```python
from build123d import *

# Parameters (mm, degrees)
SKETCH002_W    = 80.8
SKETCH002_H    = 36
PAD001_DEPTH   = 70
THICKNESS001_T = -0.8
FILLET_R       = 1
FILLET005_R    = 0.5


with BuildPart() as part:
    # Sketch002 → Pad001 (new body)
    with BuildSketch(Plane.XY):
        Rectangle(SKETCH002_W, SKETCH002_H)
    extrude(amount=PAD001_DEPTH)

    # Thickness001
    thickness001_openings = [part.faces().sort_by_distance(p)[0] for p in [
        (0, 0, 0),
    ]]
    offset(amount=THICKNESS001_T, openings=thickness001_openings, kind=Kind.INTERSECTION)

    # Fillet
    fillet_edges = [part.edges().sort_by_distance(p)[0] for p in [
        (-40.4, 18, 35),
        (-40.4, -18, 35),
        (40.4, 18, 35),
        (0, 18, 70),
        (40.4, -18, 35),
        (40.4, 0, 70),
        (0, -18, 70),
        (-40.4, 0, 70),
    ]]
    fillet(fillet_edges, radius=FILLET_R)

    # Fillet005
    fillet005_edges = [part.edges().sort_by_distance(p)[0] for p in [
        (0, -17.2, 0),
        (-39.6, 0, 0),
        (39.6, 0, 0),
        (0, 17.2, 0),
    ]]
    fillet(fillet005_edges, radius=FILLET005_R)


with BuildPart() as part_1:
    # Body001 placement: moved
    add(part.part.moved(Location((0, 0, 127))))


solid = part_1.part
```
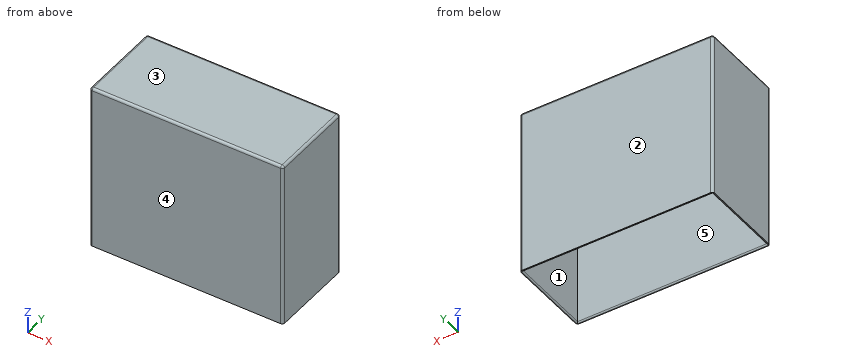
Build history of the part. All positions in model axes, mm. Face numbers are marked on the shaded views. A direction names the side the tool comes from. Round coordinates to 2 decimals unless told otherwise and drop trailing zeros. Write each loop counter-clockwise with the first axis right and the second up, starting at its lowest first coordinate (ties: lowest second). Pieces come first, ordered by that corner, then holes.
1) Pin check, flat tips, straight feed: pin 1 (6 mm diameter, centred on x = 9.5, y = 14.5, fed in from -Z); pin 2 (17 mm diameter, centred on x = -13, y = -2.5, fed in from -Z). Stop position of each tip, or through.
2) Band-saw the part on A-A, the plane y = 0. List the corners of the cut face in (x, z), and give its area (3 significant figures).
3) Mould opens along Y. For the marked faces 1, 2 and 3 say: +Y half, -Y half, draft (parallel to the pull), parting line (faces both ways), or undercut.
4) Drill centre lines: probe 1 along Y at (x, z) = (25.5, 180); probe 2 along X at (y, z) = (1, 152); probe 3 along Z at (x, y) = (2, -11). Where is each one in solid material? Low to high.
5) Band-saw the part on C-C, the plane x = -16. List the corners of the cut face in (y, z).
6) Band-saw the part on B-B, the plane z = 189. List the corners of the cut face in (x, y).
7) 3-axis set-ups, long thin cutter, end or side, ignore diameter. For the marked faces 4 and 5: which of +Z, -Z, +X, -X, +Y, -Y reach the whole face in a straight line?
Ans:
1. pin 1: stops at z = 127.04
1. pin 2: stops at z = 196.2
2. outline: (-40.4, 127) - (-40.1, 127) arc R0.5 ccw to (-39.6, 127.5) - (-39.6, 196.2) - (39.6, 196.2) - (39.6, 127.5) arc R0.5 ccw to (40.1, 127) - (40.4, 127) - (40.4, 196) arc R1 ccw to (39.4, 197) - (-39.4, 197) arc R1 ccw to (-40.4, 196) - close
2. area: 175 mm2
3. face 1: undercut
3. face 2: +Y half
3. face 3: draft
4. probe 1: y = -18 to -17.2, 17.2 to 18
4. probe 2: x = -40.4 to -39.6, 39.6 to 40.4
4. probe 3: z = 196.2 to 197
5. outline: (-18, 127) - (-17.7, 127) arc R0.5 ccw to (-17.2, 127.5) - (-17.2, 196.2) - (17.2, 196.2) - (17.2, 127.5) arc R0.5 ccw to (17.7, 127) - (18, 127) - (18, 196) arc R1 ccw to (17, 197) - (-17, 197) arc R1 ccw to (-18, 196) - close
6. outline: (-40.4, -17) arc R1 ccw to (-39.4, -18) - (39.4, -18) arc R1 ccw to (40.4, -17) - (40.4, 17) arc R1 ccw to (39.4, 18) - (-39.4, 18) arc R1 ccw to (-40.4, 17) - close; hole (-39.6, -17.2) - (39.6, -17.2) - (39.6, 17.2) - (-39.6, 17.2) - close
7. face 4: +Z, -Z, +X, -X, -Y
7. face 5: -Z
